from build123d import *

# Parameters (mm, degrees)
SKETCH1_W           = 6
SKETCH1_H           = 5
BOSS_EXTRUDE1_DEPTH = 2
SKETCH2_W           = 4
SKETCH2_H           = 2
BOSS_EXTRUDE2_DEPTH = 4
CHAMFER1_SIZE       = 1
BOSS_EXTRUDE3_DEPTH = 5
CUT_EXTRUDE1_DEPTH  = 5
SKETCH6_W           = 3
SKETCH6_H           = 2
CUT_EXTRUDE2_DEPTH  = 1


with BuildPart() as part:
    # Sketch1 → Boss-Extrude1 (new body)
    with BuildSketch(Plane(origin=(0, 0, 0), x_dir=(1, 0, 0), z_dir=(0, 1, 0))):
        Rectangle(SKETCH1_W, SKETCH1_H)
    extrude(amount=BOSS_EXTRUDE1_DEPTH)

    # Sketch2 → Boss-Extrude2 (add)
    with BuildSketch(Plane(origin=(0, 0, 0), x_dir=(1, 0, 0), z_dir=(0, 1, 0))):
        with Locations((-2, 1.5)):
            Rectangle(SKETCH2_W, SKETCH2_H)
    extrude(amount=BOSS_EXTRUDE2_DEPTH)

    # Chamfer1
    chamfer1_edges = [part.edges().sort_by_distance(p)[0] for p in [
        (-2, 4, -0.5),
    ]]
    chamfer(chamfer1_edges, length=CHAMFER1_SIZE)

    # Sketch3 → Boss-Extrude3 (add)
    with BuildSketch(Plane(origin=(0, 0, 0), x_dir=(1, 0, 0), z_dir=(0, 1, 0))):
        Polygon((3, 2.5), (5, 2.5), (5, -4.5), (4, -4.5), (4, -3.5), (3, -3.5), align=None)
    extrude(amount=BOSS_EXTRUDE3_DEPTH)

    # Sketch5 → Cut-Extrude1 (cut)
    with BuildSketch(Plane.ZY.offset(-3)):
        Polygon((-0.5, 5), (0.5, 3), (2.5, 3), (2.5, 4), (5.863314104, 4), (5.863314104, 5.536679496), align=None)
    extrude(amount=-CUT_EXTRUDE1_DEPTH, mode=Mode.SUBTRACT)

    # Sketch6 → Cut-Extrude2 (cut)
    with BuildSketch(Plane(origin=(0, 2, 0), x_dir=(1, 0, 0), z_dir=(0, 1, 0))):
        with Locations((-1.5, -1.5)):
            Rectangle(SKETCH6_W, SKETCH6_H)
    extrude(amount=-CUT_EXTRUDE2_DEPTH, mode=Mode.SUBTRACT)


solid = part.part
CAD build for the part. Positions are in the model's coordinates, mm. A direction names the side the tool comes from. Round coordinates to 2 decimals unless told otherwise and drop trailing zeros. Order: outer loops, then holes, each group sorted by start corner. A loop starts at its lowest first (then second) coordinate and runs counter-clockwise, first axis right, second up. Notation, with made-up numbers: (31, 34.5) -> (75, 34.5) arc R16 cw to (75, 54.5) -> close; hole circle Ø8 at (27.5, -35.5). An arc over 180 degrees is marked (long way). Write item = value, one per line. Start each with the question number.
(1) Cut at B-B, the plane z = -0.75. List the corners of the cut face in (x, y), then the cut area to 3 significant figures.
(2) Probe line 1 (X direction, y = 3.3, z = -1.25); line 2 (X direction, y = 2.6, z = 2.5); line 3 (Z direction, x = 1, y = 1.65). List the from-to ranges inside material, lowest first. Write a range as [from, to].
(3) Cut at A-A, the plane y = 3.3. List the corners of the cut face in (x, z).
(4) Cut at D-D, the plane x = 2.25. List the corners of the cut face in (y, z).
(5) Pin check, flat tips, straight feed: P1, Ø2, axis at y = 0.5, z = 1.5, coming from the -X side; P2, Ø0.9, axis at x = -1.5, y = 1, coming from the +Z side; P3, Ø2, axis at y = 4.5, z = 2.5, coming from the -X side; P4, Ø1.5, axis at x = -0.5, z = 0.5, coming from the -Y side. Stop position of each tip, or through.
(6) Cut at C-C, the plane y = 0.7. List the corners of the cut face in (x, z).
(7) Pull direction X, two halves, no side cores. Call faces 5 (the flat face through (5, 2, 1)), 6 (the flat face through (-2, 3.5, -1)), 7 (the flat face through (-4, 2, -1)), 8 (the flat face through (3, 2.5, 0.5)): released by +X, released by -X, zero draft, split by the parting line, or undercut.
(8) Which spindle directions (+Z, -Z, +X, -X, +Y, -Y) get a long thin tool onto all of the face, cutting with end or side? Do faces 1 (the flat face through (-2, 1, 1)), 2 (the flat face through (4, 3.5, 2.5)), 3 (the flat face through (1, 2, 0)), 4 (the flat face through (-3, 0.8, 0.7)). Say none if no direction does.
Model answer:
q1.outline = (-4, 0) -> (5, 0) -> (5, 5) -> (3, 5) -> (3, 2) -> (0, 2) -> (0, 3.25) -> (-4, 3.25) -> close
q1.area = 29.0 mm2
q2.line_1 = [-4, 0], [3, 5]
q2.line_2 = [3, 5]
q2.line_3 = [-2.5, 2.5]
q3.outline = (-4, -2.5) -> (0, -2.5) -> (0, -0.8) -> (-4, -0.8) -> close; (3, -2.5) -> (5, -2.5) -> (5, 0.35) -> (3, 0.35) -> close; (3, 2.5) -> (5, 2.5) -> (5, 4.5) -> (4, 4.5) -> (4, 3.5) -> (3, 3.5) -> close
q4.outline = (0, -2.5) -> (2, -2.5) -> (2, 2.5) -> (0, 2.5) -> close
q5.P1 = -3
q5.P2 = 2.5
q5.P3 = 3
q5.P4 = 0
q6.outline = (-4, -2.5) -> (5, -2.5) -> (5, 4.5) -> (4, 4.5) -> (4, 3.5) -> (3, 3.5) -> (3, 2.5) -> (-3, 2.5) -> (-3, -0.5) -> (-4, -0.5) -> close
q7.face_5 = released by +X
q7.face_6 = zero draft
q7.face_7 = released by -X
q7.face_8 = undercut
q8.face_1 = +Z, -X, +Y
q8.face_2 = +X, -X, +Y
q8.face_3 = +Z, +Y
q8.face_4 = +Z, -X, +Y, -Y
